For this review, take the finished solid that the model builds, in its own axes (mm). Face numbers are marked on the shaded views. A direction names the side the tool comes from. Coordinates: 2 decimals unless noted, no trailing zeros. Order: outer loops, then holes, each group sorted by start corner. A loop starts at its lowest first (then second) coordinate and runs counter-clockwise, first axis right, second up. Notation, with made-up numbers: (-32, -20) -> (-17, -20) arc R15 cw to (-17, -11) -> close; hole circle Ø4 at (54.25, 52). An arc over 180 degrees is marked (long way). Return JSON: item names as keys, results as strings. Group by question number.
Item 1: Take a section at C-C (x = 2). Write out the cut boundary in (y, z), then the cut area to 3 significant figures.
Item 2: Take a section at D-D (z = 2). Write out the cut boundary in (x, y).
Item 3: For line 1 along Y through (x, z) = (-0.25, 1); line 2 along Z through (x, y) = (1, 2.5); line 3 along Y through (x, z) = (1.25, -2), list the stretches that pass through material, from the lowest coordinate up.
Item 4: Take a section at B-B (y = 1.5). Write out the cut boundary in (x, z), then the cut area to 3 significant figures.
Item 5: Insertion check: pin 1 (3 mm diameter, centred on x = 0, z = 5.5, fed in from -Y); pin 2 (1.1 mm diameter, centred on x = 0.5, y = 3.5, fed in from +Z); pin 3 (3 mm diameter, centred on x = -1, z = 6, fed in from +Y). Each pin has a flat end and moves straight along its axis. Give the tip position at first contact, or say it passes through.
Item 6: Draft analysis for pull direction X (two halves, no side actions). For the marked faces 4, 5 and 6, state which applies: +X half, -X half, draft (parallel to the pull), parting line (faces both ways), or undercut.
Item 7: Take a section at A-A (z = -1.75). Write out the cut boundary in (x, y), then the cut area to 3 significant figures.
Item 8: Machinability: for the marked faces 1, 2 and 3, which of the approach directions +Z, -Z, +X, -X, +Y, -Y give a long, thin tool a straight path to every point of the face, cutting with its end or side? Answer none if there is none.
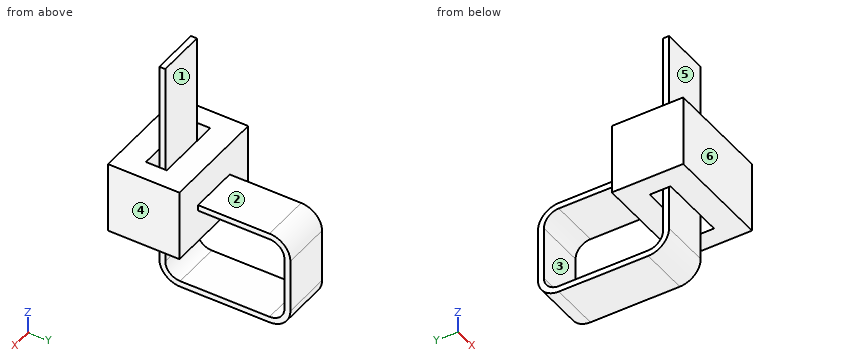
```python
from build123d import *

# Parameters (mm, degrees)
F0_W     = 5.08
F0_H     = 5.08
F1_DEPTH = 3.81
F3_W     = 3.506887937
F3_H     = 0.4214280925
F5_W     = 4.8186806962
F5_H     = 1.4827313134
F5_W_2   = 3.506887937
F5_H_2   = 0.4214280925
F6_DEPTH = 5.08


with BuildPart() as f1:
    # F0 (on Right) → F1 (new body, symmetric)
    with BuildSketch(Plane.YZ):
        Rectangle(F0_W, F0_H)
    extrude(amount=F1_DEPTH, both=True)

    # F4: sweep along a path in F2
    with BuildLine(Plane.YZ) as f4_path:
        Line((2.54, 0), (7.62, 0))
        ThreePointArc((7.62, 0), (8.5180256121, -0.3719743879), (8.89, -1.27))
        Line((8.89, -1.27), (8.89, -5.08))
        ThreePointArc((8.89, -5.08), (8.5180256121, -5.9780256121), (7.62, -6.35))
        Line((7.62, -6.35), (1.27, -6.35))
        ThreePointArc((1.27, -6.35), (0.3719743879, -5.9780256121), (0, -5.08))
        Line((0, -5.08), (0, 9.6079269424))
    # F3 (on face) → F4 (sweep)
    with BuildSketch(Plane(origin=(0, 2.54, 0), x_dir=(-1, 0, 0), z_dir=(0, 1, 0))):
        Rectangle(F3_W, F3_H)
    sweep(path=f4_path.line)

    # F5 (on face) → F6 (cut, through all)
    with BuildSketch(Plane(origin=(0, 0, -2.54), x_dir=(1, 0, 0), z_dir=(0, 0, -1))):
        Rectangle(F5_W, F5_H)
        Rectangle(F5_W_2, F5_H_2, mode=Mode.SUBTRACT)
    extrude(amount=-F6_DEPTH, mode=Mode.SUBTRACT)


solid = f1.part
```
Findings below:
{
 "1": {"outline": "(-2.54, -2.54) -> (-0.74, -2.54) -> (-0.74, 2.54) -> (-2.54, 2.54) -> close; (0.74, -2.54) -> (2.54, -2.54) -> (2.54, 2.54) -> (0.74, 2.54) -> close", "area": "18.3 mm2"},
 "2": {"outline": "(-3.81, -2.54) -> (3.81, -2.54) -> (3.81, 2.54) -> (-3.81, 2.54) -> close; (-1.75, -0.21) -> (1.75, -0.21) -> (1.75, 0.21) -> (-1.75, 0.21) -> close; hole (-2.41, -0.74) -> (2.41, -0.74) -> (2.41, 0.74) -> (-2.41, 0.74) -> close"},
 "3": {"line 1": "y = -2.54 to -0.74, -0.21 to 0.21, 0.74 to 2.54", "line 2": "z = -6.56 to -6.14, -2.54 to 2.54", "line 3": "y = -2.54 to -0.74, -0.21 to 0.21, 0.74 to 2.54, 8.68 to 9.1"},
 "4": {"outline": "(-3.81, -2.54) -> (3.81, -2.54) -> (3.81, 2.54) -> (-3.81, 2.54) -> close; (-1.75, -6.56) -> (1.75, -6.56) -> (1.75, -6.14) -> (-1.75, -6.14) -> close", "area": "40.2 mm2"},
 "5": {"pin 1": "stops at y = -0.21", "pin 2": "stops at z = 0.21", "pin 3": "stops at y = 0.21"},
 "6": {"face 4": "+X half", "face 5": "undercut", "face 6": "draft"},
 "7": {"outline": "(-3.81, -2.54) -> (3.81, -2.54) -> (3.81, 2.54) -> (-3.81, 2.54) -> close; (-1.75, -0.21) -> (1.75, -0.21) -> (1.75, 0.21) -> (-1.75, 0.21) -> close; (-1.75, 8.68) -> (1.75, 8.68) -> (1.75, 9.1) -> (-1.75, 9.1) -> close; hole (-2.41, -0.74) -> (2.41, -0.74) -> (2.41, 0.74) -> (-2.41, 0.74) -> close", "area": "34.5 mm2"},
 "8": {"face 1": "+Z", "face 2": "+Z, +X, -X, +Y", "face 3": "+X, -X"}
}
